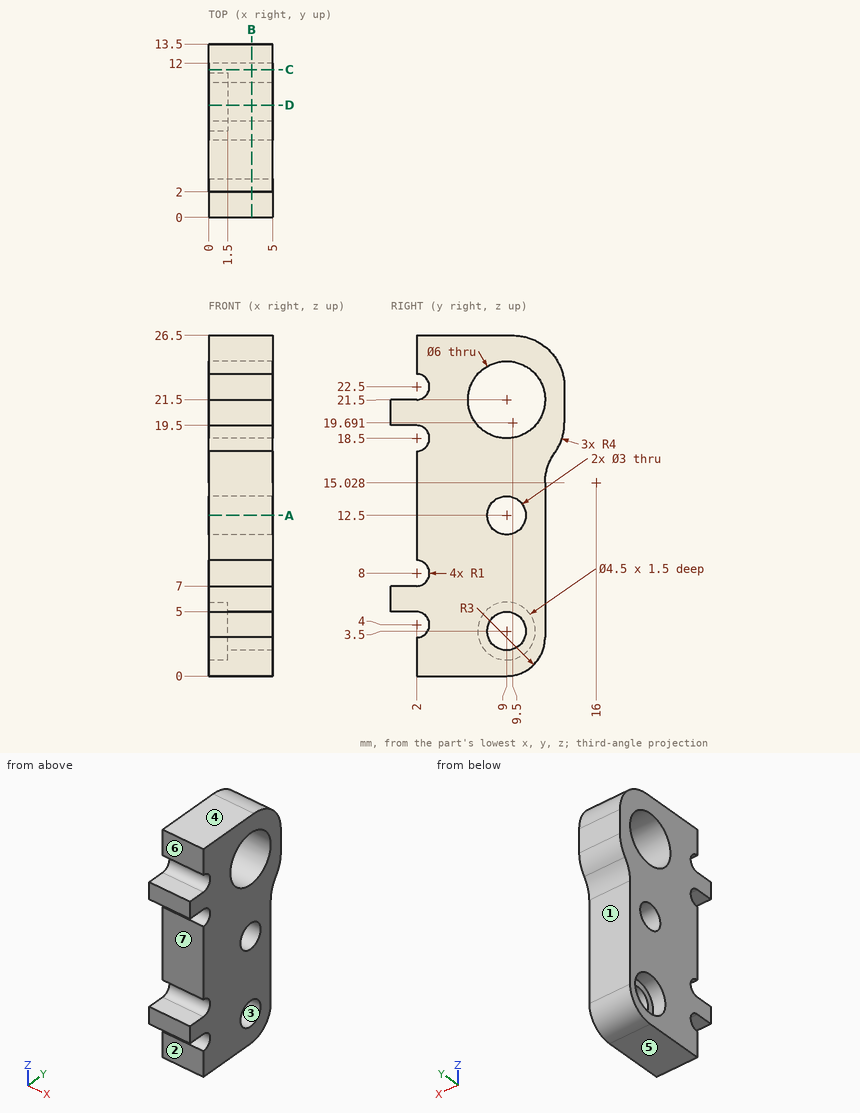
Verification items for this drawing (mm, ordinates from the low corner). A direction names the side the tool comes from. Give positions to 0.01 mm unless a question says otherwise; leave off trailing zeros. Loops run counter-clockwise (first coordinate to the right, second up) from the corner with the lowest first, then second, coordinate; pieces in that order, holes last. Notation, with made-up numbers: M 62.5,34 L 113.5,34 A32 ccw 113.5,61 Z; hole C 24.25,45 d11. An arc over 180 degrees is marked long. Return JSON: item names as keys, results as strings. Group by question number.
1. Cross-section at D-D on y = 8.75. Record the boundary of the cut face in (x, z).
2. Cross-section at C-C on y = 11.5. Record the boundary of the cut face in (x, z) (1 decimal).
3. Tool access check on the marked faces 1, 2 and 3. Record the directions out of +Z, -Z, +X, -X, +Y, -Y that give a thin tool (end or side, any length) a straight path to the whole face; none if there is none.
4. Go/stop test with flat-tipped pins: pin 1 (2.5 mm diameter, centred on y = 9, z = 12.5, fed in from +X); pin 2 (2.5 mm diameter, centred on x = 2, z = 25.5, fed in from -Y); pin 3 (1.6 mm diameter, centred on x = 3, y = 0.5, fed in from +Z); pin 4 (1 mm diameter, centred on y = 10, z = 4, fed in from -X). Record where each tip stops, or that it passes through.
5. Mould release check, pull along Z, two halves, no side actions. Record for the marked faces 4, 5, 6 and 7: released by +Z, released by -Z, zero draft, split by the parting line, or undercut.
6. Cross-section at B-B on x = 3.35. Record the boundary of the cut face in (y, z).
7. Cross-section at A-A on z = 12.5. Record the boundary of the cut face in (x, y), plus the area to 3 significant figures.
8. Thickness scan on L1, parallel to Z at x = 0.9, y = 11 (1 decimal); L2, parallel to Z at x = 4, y = 1; L3, parallel to Z at x = 1.25, y = 10 (1 decimal). Record the ranges inside material, lowest first.
Return value:
{
 "1": {"outline": "M 0,0 L 5,0 L 5,2.02 L 1.5,2.02 L 1.5,1.26 L 0,1.26 Z; M 0,5.74 L 1.5,5.74 L 1.5,4.98 L 5,4.98 L 5,11.02 L 0,11.02 Z; M 0,13.98 L 5,13.98 L 5,18.51 L 0,18.51 Z; M 0,24.49 L 5,24.49 L 5,26.5 L 0,26.5 Z"},
 "2": {"outline": "M 0,1.3 L 5,1.3 L 5,19.8 L 0,19.8 Z; M 0,23.2 L 5,23.2 L 5,26 L 0,26 Z"},
 "3": {"face 1": "-Z, +X, -X, +Y", "face 2": "-Z, +X, -X, -Y", "face 3": "+X, -X"},
 "4": {"pin 1": "through", "pin 2": "y = 2", "pin 3": "z = 21.5", "pin 4": "x = 1.5"},
 "5": {"face 4": "released by +Z", "face 5": "released by -Z", "face 6": "zero draft", "face 7": "undercut"},
 "6": {"outline": "M 0,5 L 2,5 A1 cw 2,3 L 2,0 L 9,0 A3 ccw 12,3 L 12,15.03 A4 cw 12.75,17.36 A4 ccw 13.5,19.69 L 13.5,22.5 A4 ccw 9.5,26.5 L 2,26.5 L 2,23.5 A1 cw 2,21.5 L 0,21.5 L 0,19.5 L 2,19.5 A1 cw 2,17.5 L 2,9 A1 cw 2,7 L 0,7 Z; hole C 9,21.5 d6; hole C 9,3.5 d3; hole C 9,12.5 d3"},
 "7": {"outline": "M 0,2 L 5,2 L 5,7.5 L 0,7.5 Z; M 0,10.5 L 5,10.5 L 5,12 L 0,12 Z", "area": "35.0 mm^2"},
 "8": {"L1": "0.8 to 2.5, 4.5 to 19.3, 23.7 to 26.2", "L2": "5 to 7, 19.5 to 21.5", "L3": "0.2 to 1.5, 5.5 to 11.4, 13.6 to 18.7, 24.3 to 26.5"}
}
